```python
from build123d import *

# Parameters (mm, degrees)
SKETCH1_R                       = 6.35
SKETCH1_R_2                     = 3.175
SKETCH1_R_3                     = 1.8669
EXTRUDE1_DEPTH                  = 3.175
F_4_40_TAPPED_HOLE1_D           = 2.2606
F_4_40_TAPPED_HOLE1_DEPTH       = 8.8646
F_4_40_TAPPED_HOLE1_CBORE_D     = 2.8448
F_4_40_TAPPED_HOLE1_CBORE_DEPTH = 5.6896
F_4_40_TAPPED_HOLE1_TIP         = 0.679152758
F_6_32_TAPPED_HOLE1_D           = 2.7051
F_6_32_TAPPED_HOLE1_DEPTH       = 10.922
F_6_32_TAPPED_HOLE1_TIP         = 0.81269403


with BuildPart() as part:
    # Sketch1 → Extrude1 (new body)
    with BuildSketch(Plane.XY):
        with BuildLine():
            Line((-162.56, 215.9), (162.56, 215.9))
            ThreePointArc((162.56, 215.9), (164.356051224, 215.156051224), (165.1, 213.36))
            Line((165.1, 213.36), (165.1, -213.36))
            ThreePointArc((165.1, -213.36), (164.356051224, -215.156051224), (162.56, -215.9))
            Line((162.56, -215.9), (-162.56, -215.9))
            ThreePointArc((-162.56, -215.9), (-164.356051224, -215.156051224), (-165.1, -213.36))
            Line((-165.1, -213.36), (-165.1, 213.36))
            ThreePointArc((-165.1, 213.36), (-164.356051224, 215.156051224), (-162.56, 215.9))
        make_face()
        with Locations((-149.86, 193.675)):
            Circle(SKETCH1_R, mode=Mode.SUBTRACT)
        with Locations((135.89, 193.675)):
            Circle(SKETCH1_R, mode=Mode.SUBTRACT)
        with Locations(Location((135.89, -193.675, 0), (0, 0, 180))):
            Circle(SKETCH1_R, mode=Mode.SUBTRACT)
        with Locations(Location((-149.86, -193.675, 0), (0, 0, 180))):
            Circle(SKETCH1_R, mode=Mode.SUBTRACT)
        with Locations((94.615, 142.24)):
            Circle(SKETCH1_R_2, mode=Mode.SUBTRACT)
        with Locations((94.615, 111.76)):
            Circle(SKETCH1_R_2, mode=Mode.SUBTRACT)
        with Locations((94.615, -15.24)):
            Circle(SKETCH1_R_2, mode=Mode.SUBTRACT)
        with Locations((94.615, 15.24)):
            Circle(SKETCH1_R_2, mode=Mode.SUBTRACT)
        with Locations((94.615, -142.24)):
            Circle(SKETCH1_R_2, mode=Mode.SUBTRACT)
        with Locations((94.615, -111.76)):
            Circle(SKETCH1_R_2, mode=Mode.SUBTRACT)
        with Locations((53.34, 177.8)):
            Circle(SKETCH1_R_3, mode=Mode.SUBTRACT)
        with Locations((-99.06, 177.8)):
            Circle(SKETCH1_R_3, mode=Mode.SUBTRACT)
    extrude(amount=EXTRUDE1_DEPTH)

    # #4-40 Tapped Hole1
    with Locations(Plane.XY.offset(3.175)):
        with Locations((-147.32, 113.665), (-43.18, 113.665), (-43.18, -41.275), (-147.32, -41.275), (-118.745, -85.09), (0.635, -85.09), (97.79, -85.09), (97.79, -199.39), (0.635, -199.39), (-118.745, -199.39), (-121.92, 113.665), (-17.78, 113.665), (-17.78, -41.275), (-121.92, -41.275), (17.451090556, 117.318318975), (68.251090556, 117.318318975), (119.051090556, 117.318318975), (17.451090556, 79.218318975), (17.451090556, 41.118318975), (68.251090556, 79.218318975), (119.051090556, 79.218318975), (119.051090556, 41.118318975), (68.251090556, 41.118318975), (17.451090556, 3.018318975), (68.251090556, 3.018318975), (119.051090556, 3.018318975), (119.051090556, -35.081681025), (68.251090556, -35.081681025), (17.451090556, -35.081681025)):
            CounterBoreHole(F_4_40_TAPPED_HOLE1_D / 2, F_4_40_TAPPED_HOLE1_CBORE_D / 2, F_4_40_TAPPED_HOLE1_CBORE_DEPTH, depth=F_4_40_TAPPED_HOLE1_DEPTH)
            with Locations((0, 0, -(F_4_40_TAPPED_HOLE1_DEPTH + F_4_40_TAPPED_HOLE1_TIP / 2))):  # 118° drill point
                Cone(0, F_4_40_TAPPED_HOLE1_D / 2, F_4_40_TAPPED_HOLE1_TIP, mode=Mode.SUBTRACT)

    # #6-32 Tapped Hole1
    with Locations(Plane.XY.offset(3.175)):
        with Locations((59.69, 171.45), (-105.41, 171.45)):
            Hole(F_6_32_TAPPED_HOLE1_D / 2, depth=F_6_32_TAPPED_HOLE1_DEPTH)
            with Locations((0, 0, -(F_6_32_TAPPED_HOLE1_DEPTH + F_6_32_TAPPED_HOLE1_TIP / 2))):  # 118° drill point
                Cone(0, F_6_32_TAPPED_HOLE1_D / 2, F_6_32_TAPPED_HOLE1_TIP, mode=Mode.SUBTRACT)


solid = part.part
```
Read the model definition and answer for the solid it produces. Units are mm, in the model's axes. Give positions to 0.01 mm unless a question says otherwise; leave off trailing zeros. Write each loop counter-clockwise with the first axis right and the second up, starting at its lowest first coordinate (ties: lowest second). Pieces come first, ordered by that corner, then holes. Notation, with made-up numbers: M -31.5,85 L 12.5,85 A13 cw 12.5,95 Z; hole C -19,57 d9. An arc over 180 degrees is marked long. Put each result on its own line as item: value. Start each with the question number.
1. Consider line 1 along Y through (x, z) = (135, 1.05); line 2 along Y through (x, z) = (98, 0.6); line 3 along X through (y, z) = (171.45, 2.5). Determine where each line is inside the solid, lowest interval first.
2. The part is cut by section A-A, the plane x = 135.89. Give the vertices of the cut face in (y, z) (3 decimals), and give its area (3 significant figures).
3. This flat-tipped pin is pushed along its axis until it touches: pin 1 Ø2.5 at (x, y) = (17.45, 3.02) entering from -Z. Where does it stop, or does it pass through?
4. For a pull along Y with two mould halves and no side action, classify faces 1 (the cylindrical face through (-148.483, -187.476, 1.565)), 2 (the flat face through (2, 3, 0)) as released by +Y, released by -Y, zero draft, split by the parting line, or undercut.
Final values:
1. line 1: y = -215.9 to -199.96, -187.39 to 187.39, 199.96 to 215.9
1. line 2: y = -215.9 to -200.8, -197.98 to -86.5, -83.68 to 215.9
1. line 3: x = -165.1 to -106.76, -104.06 to 58.34, 61.04 to 165.1
2. outline: M -215.9,0 L -200.025,0 L -200.025,3.175 L -215.9,3.175 Z; M -187.325,0 L 187.325,0 L 187.325,3.175 L -187.325,3.175 Z; M 200.025,0 L 215.9,0 L 215.9,3.175 L 200.025,3.175 Z
2. area: 1,290 mm²
3. pin 1: passes through
4. face 1: undercut
4. face 2: zero draft
